from build123d import *

# Parameters (mm, degrees)
BOSS_EXTRUDE1_DEPTH              = 304.800275
FILLET1_R                        = 8
CUT_EXTRUDE1_REACH               = 6.806
CUT_EXTRUDE1_OFFSET_FROM_SURFACE = 1
SKETCH2_W                        = 38.10085
SKETCH2_H                        = 23.904524524
SKETCH2_W_2                      = 38.1
FILLET2_R                        = 1.6
FILLET3_R                        = 1.6


with BuildPart() as part:
    # Sketch1 → Boss-Extrude1 (new body)
    with BuildSketch(Plane.ZY.offset(149.225)):
        Polygon((-2, -64.023653), (-3.3962, -64.023653), (-3.3962, -50.048837521), (-4.3962, -50.048837521), (-4.3962, -28.126347), (-5.3962, -28.126347), (-5.3962, 3.873653), (-7.3962, 3.873653), (-7.3962, 29.378177524), (-11.202667042, 29.378177524), (-4, -73.62476), (-2, -73.62476), align=None)
    extrude(amount=-BOSS_EXTRUDE1_DEPTH)

    # Fillet1
    fillet1_edges = [part.edges().sort_by_distance(p)[0] for p in [
        (-149.225, 29.378177524, -9.299433521),
        (155.575275, 29.378177524, -9.299433521),
    ]]
    fillet(fillet1_edges, radius=FILLET1_R)

    # Cut-Extrude1: up to this face of the body (flat: up to its plane, moved by the offset)
    cut_extrude1_end = Plane(part.part.faces().sort_by_distance((3.1751375, -22.166826572, -7.598289234))[0]).offset(-CUT_EXTRUDE1_OFFSET_FROM_SURFACE)
    # Sketch2 → Cut-Extrude1 (cut, up to the picked face)
    with BuildSketch(Plane.XY.offset(-7.3962), mode=Mode.PRIVATE) as cut_extrude1_sk1:
        with Locations((41.2757, 17.425915262)):
            Rectangle(SKETCH2_W, SKETCH2_H)
    cut_extrude1_tool1 = split(extrude(cut_extrude1_sk1.sketch, amount=-CUT_EXTRUDE1_REACH, mode=Mode.PRIVATE), bisect_by=cut_extrude1_end, keep=Keep.BOTH, mode=Mode.PRIVATE)
    add(cut_extrude1_tool1.solids().sort_by_distance((41.2757, 17.425915, -7.3962))[0], mode=Mode.SUBTRACT)
    # Sketch2 → Cut-Extrude1 (cut, up to the picked face)
    with BuildSketch(Plane.XY.offset(-7.3962), mode=Mode.PRIVATE) as cut_extrude1_sk2:
        with Locations((-92.074875, 17.425915262)):
            Rectangle(SKETCH2_W_2, SKETCH2_H)
    cut_extrude1_tool2 = split(extrude(cut_extrude1_sk2.sketch, amount=-CUT_EXTRUDE1_REACH, mode=Mode.PRIVATE), bisect_by=cut_extrude1_end, keep=Keep.BOTH, mode=Mode.PRIVATE)
    add(cut_extrude1_tool2.solids().sort_by_distance((-92.074875, 17.425915, -7.3962))[0], mode=Mode.SUBTRACT)
    # Sketch2 → Cut-Extrude1 (cut, up to the picked face)
    with BuildSketch(Plane.XY.offset(-7.3962), mode=Mode.PRIVATE) as cut_extrude1_sk3:
        with Locations((-34.92515, 17.425915262)):
            Rectangle(SKETCH2_W, SKETCH2_H)
    cut_extrude1_tool3 = split(extrude(cut_extrude1_sk3.sketch, amount=-CUT_EXTRUDE1_REACH, mode=Mode.PRIVATE), bisect_by=cut_extrude1_end, keep=Keep.BOTH, mode=Mode.PRIVATE)
    add(cut_extrude1_tool3.solids().sort_by_distance((-34.92515, 17.425915, -7.3962))[0], mode=Mode.SUBTRACT)
    # Sketch2 → Cut-Extrude1 (cut, up to the picked face)
    with BuildSketch(Plane.XY.offset(-7.3962), mode=Mode.PRIVATE) as cut_extrude1_sk4:
        with Locations((98.425425, 17.425915262)):
            Rectangle(SKETCH2_W_2, SKETCH2_H)
    cut_extrude1_tool4 = split(extrude(cut_extrude1_sk4.sketch, amount=-CUT_EXTRUDE1_REACH, mode=Mode.PRIVATE), bisect_by=cut_extrude1_end, keep=Keep.BOTH, mode=Mode.PRIVATE)
    add(cut_extrude1_tool4.solids().sort_by_distance((98.425425, 17.425915, -7.3962))[0], mode=Mode.SUBTRACT)

    # Fillet2
    fillet2_edges = [part.edges().sort_by_distance(p)[0] for p in [
        (-73.024875, 5.473653, -7.962428976),
        (-111.124875, 5.473653, -7.962428976),
        (-15.874725, 5.473653, -7.962428976),
        (-53.975575, 5.473653, -7.962428976),
        (22.225275, 5.473653, -7.962428976),
        (60.326125, 5.473653, -7.962428976),
        (79.375425, 5.473653, -7.962428976),
        (117.475425, 5.473653, -7.962428976),
    ]]
    fillet(fillet2_edges, radius=FILLET2_R)

    # Fillet3
    fillet3_edges = [part.edges().sort_by_distance(p)[0] for p in [
        (-73.024875, 29.378177524, -8.798212572),
        (-111.124875, 29.378177524, -8.798212572),
        (-15.874725, 29.378177524, -8.798212572),
        (-53.975575, 29.378177524, -8.798212572),
        (60.326125, 29.378177524, -8.798212572),
        (22.225275, 29.378177524, -8.798212572),
        (117.475425, 29.378177524, -8.798212572),
        (79.375425, 29.378177524, -8.798212572),
    ]]
    fillet(fillet3_edges, radius=FILLET3_R)


solid = part.part
Could you check a few things on this model? Use its own coordinates, in mm. A direction names the side the tool comes from. Coordinates: 2 decimals unless noted, no trailing zeros. Order: outer loops, then holes, each group sorted by start corner. A loop starts at its lowest first (then second) coordinate and runs counter-clockwise, first axis right, second up.
Q1. Thinking about a two-plate mould opening in X: for faces 1 (the flat face through (1, -69, -2)), 2 (the cylindrical face through (-146.819, 27.097, -9.326)), 3 (the flat face through (-92.364, 17.593, -9.376)), which applies, released by +X, released by -X, zero draft, split by the parting line, or undercut?
Q2. Which directions (+Z, -Z, +X, -X, +Y, -Y) give clear straight access to the entire face, cutting with the end or side of a thin tool? Please do faces 4 (the flat face through (-35.214, 17.593, -9.376)), 5 (the flat face through (-149.225, -22, -7)), 6 (the flat face through (1, -57, -3.396)).
Q3. Suppose I cut it at D-D on y = -9. Please give me the cut outline in (x, z) (3 decimals).
Q4. Will these pins go through, and if not, where does the flat tip stop? pin 1 (1.5 mm diameter, centred on x = 78.5, y = -43.5, fed in from -Z); pin 2 (0.7 mm diameter, centred on x = 69.5, z = -2.5, fed in from +Y); pin 3 (0.8 mm diameter, centred on y = 22, z = -8, fed in from -X); pin 4 (1 mm diameter, centred on y = -30.5, z = -9.5, fed in from -X).
Q5. Please list where these lines run through material, in increasing order: L1, parallel to Z at x = -27, y = -6.5; L2, parallel to Z at x = -9, y = 13.5.
Q6. Suppose I cut it at A-A on x = -60.5. Please give me the cut outline in (y, z).
Q7. Suppose I cut it at B-B on x = -97. Please give me the cut outline in (y, z), and give its area (3 significant figures).
Q8. Suppose I cut it at C-C on y = -54. Please give me the cut outline in (x, z) (3 decimals).
Answer:
1. face 1: zero draft
1. face 2: released by -X
1. face 3: undercut
2. face 4: +Z, +Y
2. face 5: +Z, -Z, -X, +Y, -Y
2. face 6: +Z, +X, -X, +Y
3. outline: (-149.225, -8.519) - (155.575, -8.519) - (155.575, -5.396) - (-149.225, -5.396) - close
4. pin 1: stops at z = -6.16
4. pin 2: stops at y = -64.02
4. pin 3: stops at x = -149.22
4. pin 4: passes through
5. L1: z = -8.69 to -5.4
5. L2: z = -10.09 to -7.4
6. outline: (-73.62, -4) - (29.38, -11.2) - (29.38, -7.4) - (3.87, -7.4) - (3.87, -5.4) - (-28.13, -5.4) - (-28.13, -4.4) - (-50.05, -4.4) - (-50.05, -3.4) - (-64.02, -3.4) - (-64.02, -2) - (-73.62, -2) - close
7. outline: (-73.62, -4) - (29.38, -11.2) - (29.38, -10.2) - (5.47, -8.53) - (5.47, -7.4) - (3.87, -7.4) - (3.87, -5.4) - (-28.13, -5.4) - (-28.13, -4.4) - (-50.05, -4.4) - (-50.05, -3.4) - (-64.02, -3.4) - (-64.02, -2) - (-73.62, -2) - close
7. area: 212 mm2
8. outline: (-149.225, -5.372) - (155.575, -5.372) - (155.575, -3.396) - (-149.225, -3.396) - close
